The listing builds one solid part. Answer for the finished solid, in the listing's coordinates (mm). A direction names the side the tool comes from. Give positions to 0.01 mm unless a question says otherwise; leave off trailing zeros. Write each loop counter-clockwise with the first axis right and the second up, starting at its lowest first coordinate (ties: lowest second). Pieces come first, ordered by that corner, then holes. Notation, with made-up numbers: (31, 2) - (46, 2) arc R7 ccw to (46, 14) - close; hole circle Ø1 at (-19.75, 73). An arc over 180 degrees is marked (long way). One line per question, with ' | ' between items. Start each with the question number.
1. For faces 1 (the face through (13.66, 0.99, -11.26)), 2 (the face through (12, 2, -5)), determine the directions among +Z, -Z, +X, -X, +Y, -Y from which every point of the face is accessible in a straight line to the end or side of a thin tool.
2. Given P1, Ø5, axis at y = 15.5, z = 6.5, coming from the -X side; P2, Ø10, axis at x = -3.5, y = 14.5, coming from the -Z side; P3, Ø3, axis at x = 12.52, z = -12.52, coming from the -Y side; P4, Ø3, axis at y = 7.5, z = -3, coming from the -X side, each flat-ended and moving along its own axis, determine where each tip first touches the part or whether it passes through.
3. Find the intervals of material crossed by L1, parallel to Z at x = 0.5, y = 12.5; L2, parallel to Y at x = 14.5, z = -11.5; L3, parallel to X at y = 6.25, z = 5, in increasing order. Write a range as from..to.
4. A cutting plane is placed at A-A (x = 0). Determine the outline of the cut face in (y, z).
5. A cutting plane is placed at C-C (y = 7). Determine the outline of the cut face in (x, z), then the cut area to 3 significant figures.
6. A cutting plane is placed at D-D (x = -13.5). Determine the outline of the cut face in (y, z).
7. The mould has two halves that part along Z. Classify faces 3 (the face through (-13.55, 0.986, -11.167)), 4 (the face through (12.274, 10.406, 2.726)), 5 (the face through (-17.78, 1, 0)): +Z half, -Z half, draft (parallel to the pull), parting line (faces both ways), or undercut.
8. A cutting plane is placed at B-B (z = 0). Determine the outline of the cut face in (x, y).
```python
from build123d import *

# Parameters (mm, degrees)
CUT_EXTRUDE2_DEPTH       = 35.926816345
M3_CLEARANCE_HOLE1_D     = 3.4
M3_CLEARANCE_HOLE1_DEPTH = 12.7


with BuildPart() as part:
    # Sketch1 → Revolve1 (revolve)
    with BuildSketch(Plane.XY, mode=Mode.PRIVATE) as revolve1_sk:
        Polygon((12.573, 2), (20.7, 2), (20.7, 0), (11.073, 0), (11.073, 19.05), (12.573, 19.05), align=None)
    revolve(revolve1_sk.sketch.rotate(Axis((0, 0, 0), (0, 1, 0)), 90), axis=Axis((0, 0, 0), (0, 1, 0)))

    # Sketch3 → Cut-Extrude2 (cut, through all)
    with BuildSketch(Plane.XZ):
        with BuildLine():
            Line((-17.78, 10.600075471), (-17.78, -10.600075471))
            ThreePointArc((-17.78, -10.600075471), (-20.7, 0), (-17.78, 10.600075471))
        make_face()
        with BuildLine():
            Line((17.78, -10.600075471), (17.78, 10.600075471))
            ThreePointArc((17.78, 10.600075471), (20.7, 0), (17.78, -10.600075471))
        make_face()
    extrude(amount=-CUT_EXTRUDE2_DEPTH, mode=Mode.SUBTRACT)

    # M3 Clearance Hole1
    with Locations(Plane(origin=(12.515790027, 2, 12.515790027), x_dir=(0, 0, 1), z_dir=(0, 1, 0))):
        with Locations((0, 0), (0, -25.031580054), (-25.031580054, -25.031580054), (-25.031580054, 0)):
            Hole(M3_CLEARANCE_HOLE1_D / 2, depth=M3_CLEARANCE_HOLE1_DEPTH)


solid = part.part
```
Determined:
1) face 1: +Y, -Y | face 2: +Y
2) P1: x = -11.92 | P2: z = -12.57 | P3: through | P4: x = -12.48
3) L1: -12.56..-11.06, 11.06..12.56 | L2: 0..2 | L3: -11.54..-9.88, 9.88..11.54
4) outline: (0, -20.7) - (2, -20.7) - (2, -12.57) - (19.05, -12.57) - (19.05, -11.07) - (0, -11.07) - close; (0, 11.07) - (19.05, 11.07) - (19.05, 12.57) - (2, 12.57) - (2, 20.7) - (0, 20.7) - close
5) outline: circle Ø25.15 at (0, 0); hole circle Ø22.15 at (0, 0) | area: 111 mm2
6) outline: (0, -15.69) - (2, -15.69) - (2, -13.9) - (0, -13.9) - close; (0, -11.13) - (2, -11.13) - (2, 11.13) - (0, 11.13) - close; (0, 13.9) - (2, 13.9) - (2, 15.69) - (0, 15.69) - close
7) face 3: undercut | face 4: parting line | face 5: draft
8) outline: (-17.78, 0) - (-11.07, 0) - (-11.07, 19.05) - (-12.57, 19.05) - (-12.57, 2) - (-17.78, 2) - close; (11.07, 0) - (17.78, 0) - (17.78, 2) - (12.57, 2) - (12.57, 19.05) - (11.07, 19.05) - close
